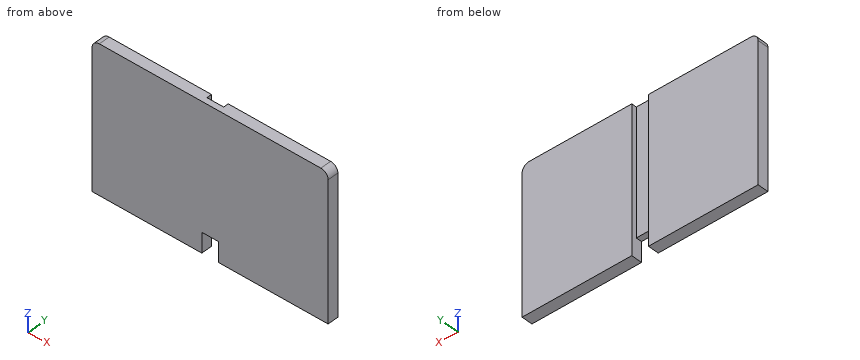
Autodesk Fusion 360 part; units mm, degrees
sketch "Skizze1" plane through (0, 0, 0) normal (0, 1, 0) x (1, 0, 0)
  line L0 (32.5, 20) -> (-32.5, 20)
  line L1 (-32.5, 20) -> (-32.5, -20)
  line L2 (-32.5, -20) -> (32.5, -20)
  line L3 (32.5, -20) -> (32.5, 20)
  line L4 (32.5, 20) -> (-32.5, -20) construction
  line L5 (-32.5, 20) -> (32.5, -20) construction
  dimension "d1" = 40
  dimension "d2" = 65
extrude "Extrusion1" add sketch "Skizze1" along normal blind 3
sketch "Skizze2" plane through (0, 3, 0) normal (0, 1, 0) x (-1, 0, 0)
  line L0 (-32.5, 20) -> (-32.5, -20)
  line L1 (-32.5, -20) -> (32.5, -20)
  line L2 (32.5, -20) -> (32.5, 20)
  line L3 (32.5, 20) -> (-32.5, 20)
  line L4 (2.3, -20) -> (-2.3, -20)
  line L5 (-2.3, -20) -> (-2.3, -14.5)
  line L6 (-2.3, -14.5) -> (2.3, -14.5)
  line L7 (2.3, -14.5) -> (2.3, -20)
  line L8 (2.3, -20) -> (-2.3, -14.5) construction
  line L9 (-2.3, -20) -> (2.3, -14.5) construction
  point P0 (0, -17.25)
  dimension "d5" = 4.6
  dimension "d6" = 5.5
extrude "Extrusion2" cut sketch "Skizze2" against normal blind 3 contours L1 L4 L5 L6 L7
sketch "Skizze3" plane through (0, 3, 0) normal (0, 1, 0) x (-1, 0, 0)
  line L0 (2.3, -14.5) -> (2.3, -20)
  line L1 (2.3, -20) -> (32.5, -20)
  line L2 (32.5, -20) -> (32.5, 20)
  line L3 (32.5, 20) -> (-32.5, 20)
  line L4 (-32.5, 20) -> (-32.5, -20)
  line L5 (-32.5, -20) -> (-2.3, -20)
  line L6 (-2.3, -20) -> (-2.3, -14.5)
  line L7 (-2.3, -14.5) -> (2.3, -14.5)
  line L8 (2.3, -14.5) -> (-2.3, -14.5)
  line L9 (-2.3, -14.5) -> (-2.3, 20)
  line L10 (-2.3, 20) -> (2.3, 20)
  line L11 (2.3, 20) -> (2.3, -14.5)
extrude "Extrusion3" cut sketch "Skizze3" against normal blind 1.4 contours L3 L7 L8 L9 L10 L11
fillet "Abrundung1" radius 2 2 edges at (-32.5, 1.5, 20) (32.5, 1.5, 20)
Input: part model. Units: mm. Frame: model coordinates. Give positions to 0.01 mm unless a question says otherwise; leave off trailing zeros. Loops run counter-clockwise (first coordinate to the right, second up) from the corner with the lowest first, then second, coordinate; pieces in that order, holes last. Notation, with made-up numbers: M 72.25,18.5 L 86.25,18.5 A33 cw 86.25,50.5 Z; hole C -36.75,-8.75 d2. An arc over 180 degrees is marked long. Answer as CSV lines item,"result". Start each with the question number.
1. Section A-A on z = -17. Return loops of the section in (x, y).
2. Section D-D on x = 1. Return loops of the section in (y, z).
3. Pin query (flat end, axial travel): P1, Ø0.5, axis at x = 1, y = 1, coming from the -Z side. Return the tip coordinate at first contact, or that it passes through.
4. Line query: L1, parallel to X at y = 2.2, z = 7; L2, parallel to Y at x = -1, z = 13. Output: solid intervals per line, ascending.
5. Section C-C on z = 8.5. Return loops of the section in (x, y).
6. Section B-B on y = 2.55. Return loops of the section in (x, z).
Computed values:
1,outline,"M -32.5,0 L -2.3,0 L -2.3,3 L -32.5,3 Z; M 2.3,0 L 32.5,0 L 32.5,3 L 2.3,3 Z"
2,outline,"M 0,-14.5 L 1.6,-14.5 L 1.6,20 L 0,20 Z"
3,P1,"stops at z = -14.5"
4,L1,"x = -32.5 to -2.3, 2.3 to 32.5"
4,L2,"y = 0 to 1.6"
5,outline,"M -32.5,0 L 32.5,0 L 32.5,3 L 2.3,3 L 2.3,1.6 L -2.3,1.6 L -2.3,3 L -32.5,3 Z"
6,outline,"M -32.5,-20 L -2.3,-20 L -2.3,20 L -30.5,20 A2 ccw -32.5,18 Z; M 2.3,-20 L 32.5,-20 L 32.5,18 A2 ccw 30.5,20 L 2.3,20 Z"
